Design review of the part built by this model. Coordinates are the model's own, in mm. Face numbers are marked on the shaded views. A direction names the side the tool comes from. Coordinates: 2 decimals unless noted, no trailing zeros. Loops run counter-clockwise (first coordinate to the right, second up) from the corner with the lowest first, then second, coordinate; pieces in that order, holes last. Notation, with made-up numbers: M 36,44 L 52,44 A8 ccw 52,57 Z; hole C -33.75,46 d4. An arc over 180 degrees is marked long. Write item = value, one per line. Start each with the question number.
from build123d import *

# Parameters (mm, degrees)
ESBO_O1_W                = 5
ESBO_O1_H                = 15
RESSALTO_EXTRUS_O1_DEPTH = 3.6
ESBO_O2_W                = 3
ESBO_O2_H                = 15
CORTE_EXTRUS_O2_DEPTH    = 3
ESBO_O3_W                = 1.2
ESBO_O3_H                = 13
CORTE_EXTRUS_O3_DEPTH    = 17.21604144


with BuildPart() as part:
    # Esboço1 → Ressalto-extrusão1 (new body)
    with BuildSketch(Plane(origin=(0, 0, 0), x_dir=(1, 0, 0), z_dir=(0, 1, 0))):
        with Locations((-2.5, 7.5)):
            Rectangle(ESBO_O1_W, ESBO_O1_H)
    extrude(amount=RESSALTO_EXTRUS_O1_DEPTH)

    # Esboço2 → Corte-extrusão2 (cut)
    with BuildSketch(Plane(origin=(0, 3.6, 0), x_dir=(1, 0, 0), z_dir=(0, 1, 0))):
        with Locations((-1.5, 7.5)):
            Rectangle(ESBO_O2_W, ESBO_O2_H)
    extrude(amount=-CORTE_EXTRUS_O2_DEPTH, mode=Mode.SUBTRACT)

    # Esboço3 → Corte-extrusão3 (cut, through all)
    with BuildSketch(Plane(origin=(0, 3.6, 0), x_dir=(1, 0, 0), z_dir=(0, 1, 0))):
        with Locations((-3.6, 7.5)):
            Rectangle(ESBO_O3_W, ESBO_O3_H)
    extrude(amount=-CORTE_EXTRUS_O3_DEPTH, mode=Mode.SUBTRACT)


solid = part.part
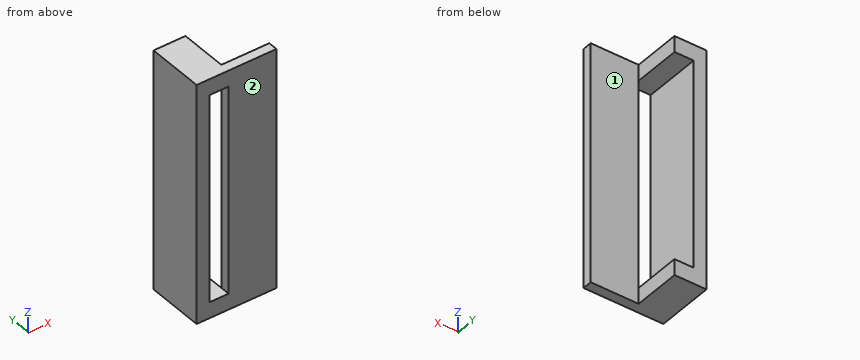
Q1. Clearance check with flat-ended pins moving along their axes: P1, Ø1.1, axis at y = 1.5, z = -7, coming from the +X side; P2, Ø0.8, axis at y = 1.5, z = -0.5, coming from the +X side. State where each tip first meets the part, or that it passes through.
Q2. Add section B-B on y = 0.45. State the section outline as (x, z) points, plus the area to 3 significant figures.
Q3. For the marked faces 1 and 2, list the 3-axis set-ups (+Z, -Z, +X, -X, +Y, -Y) from which the entire face can be reached by the end or side of a thin tool; tool diameter is ignored.
Q4. To check wall thickness, follow line 1 (X direction, y = 0.25, z = -10); line 2 (X direction, y = 0.65, z = -10.75); line 3 (Y direction, x = -1.7, z = -11.75). State the ranges of each line that lie inside material, in increasing order. Write a range as from..to.
Q5. Add section D-D on y = 2. State the section outline as (x, z) points.
Q6. Add section A-A on z = -2.25. State the section outline as (x, y) points, plus the area to 3 significant figures.
Q7. Add section C-C on x = -3.7. State the section outline as (y, z) points, plus the area to 3 significant figures.
Values follow:
q1.P1 = -4.2
q1.P2 = -3
q2.outline = M -5,-15 L 0,-15 L 0,0 L -5,0 Z; hole M -4.2,-14 L -3,-14 L -3,-1 L -4.2,-1 Z
q2.area = 59.4 mm2
q3.face_1 = +Z, -Z, +X, +Y
q3.face_2 = +Z, -Z, +X, -X, -Y
q4.line_1 = -5..-4.2, -3..0
q4.line_2 = -5..-4.2
q4.line_3 = 0..0.6
q5.outline = M -5,-15 L -3,-15 L -3,-14 L -4.2,-14 L -4.2,-1 L -3,-1 L -3,0 L -5,0 Z
q6.outline = M -5,0 L -4.2,0 L -4.2,3.6 L -5,3.6 Z; M -3,0 L 0,0 L 0,0.6 L -3,0.6 Z
q6.area = 4.68 mm2
q7.outline = M 0,-15 L 3.6,-15 L 3.6,-14 L 0,-14 Z; M 0,-1 L 3.6,-1 L 3.6,0 L 0,0 Z
q7.area = 7.20 mm2
